Work out the finished part from the listing and answer in its coordinate system (mm). A direction names the side the tool comes from. Coordinates: 2 decimals unless noted, no trailing zeros. Write each loop counter-clockwise with the first axis right and the second up, starting at its lowest first coordinate (ties: lowest second). Pieces come first, ordered by that corner, then holes. Notation, with made-up numbers: (0.25, 14) - (26.25, 14) arc R18 cw to (26.25, 18) - close; hole circle Ø9 at (-24.5, 40.5). An arc over 180 degrees is marked (long way). One line per item, written item: value.
```python
from build123d import *

# Parameters (mm, degrees)
SKETCH1_W           = 18
SKETCH1_H           = 50
BOSS_EXTRUDE1_DEPTH = 3
SKETCH2_W           = 3
SKETCH2_H           = 15
BOSS_EXTRUDE2_DEPTH = 15
SKETCH3_R           = 1.65
CUT_EXTRUDE1_DEPTH  = 3


with BuildPart() as part:
    # Sketch1 → Boss-Extrude1 (new body)
    with BuildSketch(Plane(origin=(0, 0, 0), x_dir=(1, 0, 0), z_dir=(0, 1, 0))):
        Rectangle(SKETCH1_W, SKETCH1_H)
    extrude(amount=BOSS_EXTRUDE1_DEPTH)

    # Sketch2 → Boss-Extrude2 (add)
    with BuildSketch(Plane(origin=(0, 3, 0), x_dir=(1, 0, 0), z_dir=(0, 1, 0))):
        with Locations((7.5, 17.5)):
            Rectangle(SKETCH2_W, SKETCH2_H)
        with Locations((-7.5, 17.5)):
            Rectangle(SKETCH2_W, SKETCH2_H)
        with Locations((-7.5, -17.5)):
            Rectangle(SKETCH2_W, SKETCH2_H)
        with Locations((7.5, -17.5)):
            Rectangle(SKETCH2_W, SKETCH2_H)
    extrude(amount=BOSS_EXTRUDE2_DEPTH)

    # Sketch3 → Cut-Extrude1 (cut)
    with BuildSketch(Plane.XZ):
        with Locations(Location((0, 15, 0), (0, 0, 270))):
            Circle(SKETCH3_R)
        with Locations(Location((0, -15, 0), (0, 0, 90))):
            Circle(SKETCH3_R)
    extrude(amount=-CUT_EXTRUDE1_DEPTH, mode=Mode.SUBTRACT)


solid = part.part
```
Item 1: Which of the six approach directions +Z, -Z, +X, -X, +Y, -Y give full straight-line access (tool end or side, diameter ignored) to faces 1 (the face through (9, 1, 0)), 2 (the face through (-8, 10, 10)), 3 (the face through (-6, 10, -17))?
Evaluation:
face 1: +Z, -Z, +X, +Y, -Y
face 2: +X, -X, +Y
face 3: +Z, -Z, +Y
Item 2: Section B-B, the plane z = -15 is taken. Determine the outline of the cut face in (x, y).
Evaluation:
outline: (-9, 0) - (-1.65, 0) - (-1.65, 3) - (-6, 3) - (-6, 18) - (-9, 18) - close; (1.65, 0) - (9, 0) - (9, 18) - (6, 18) - (6, 3) - (1.65, 3) - close
Item 3: Section A-A, the plane y = 10.5 is taken. Determine the outline of the cut face in (x, z).
Evaluation:
outline: (-9, -25) - (-6, -25) - (-6, -10) - (-9, -10) - close; (-9, 10) - (-6, 10) - (-6, 25) - (-9, 25) - close; (6, -25) - (9, -25) - (9, -10) - (6, -10) - close; (6, 10) - (9, 10) - (9, 25) - (6, 25) - close
Item 4: Determine the mould class of faces 4 (the face through (-9, 1, 0)), 5 (the face through (0, 0, 0)), 6 (the face through (-6, 10, 18)) for opening direction X: +X half, -X half, draft (parallel to the pull), parting line (faces both ways), or undercut.
Evaluation:
face 4: -X half
face 5: draft
face 6: undercut
Item 5: Given pin 1 (5 mm diameter, centred on x = 0.5, z = -16.5, fed in from +Y); pin 2 (3 mm diameter, centred on x = 0, z = 15, fed in from -Y) (3 decimals), each flat-ended and moving along its own axis, determine where each tip first touches the part or whether it passes through.
Evaluation:
pin 1: stops at y = 3
pin 2: passes through
Item 6: Consider probe 1 along X at (y, z) = (2.3, -15); probe 2 along X at (y, z) = (14.5, -17); probe 3 along Z at (x, y) = (-6.5, 15). Determine where each line is inside the solid, lowest interval first.
Evaluation:
probe 1: x = -9 to -1.65, 1.65 to 9
probe 2: x = -9 to -6, 6 to 9
probe 3: z = -25 to -10, 10 to 25
Item 7: Section C-C, the plane x = 0 is taken. Determine the outline of the cut face in (y, z).
Evaluation:
outline: (0, -25) - (3, -25) - (3, -16.65) - (0, -16.65) - close; (0, -13.35) - (3, -13.35) - (3, 13.35) - (0, 13.35) - close; (0, 16.65) - (3, 16.65) - (3, 25) - (0, 25) - close
Item 8: Section D-D, the plane z = 19 is taken. Determine the outline of the cut face in (x, y).
Evaluation:
outline: (-9, 0) - (9, 0) - (9, 18) - (6, 18) - (6, 3) - (-6, 3) - (-6, 18) - (-9, 18) - close
